from build123d import *

# Parameters (mm, degrees)
CUT_EXTRUDE1_DEPTH = 10
CIRPATTERN1_COUNT  = 20


with BuildPart() as part:
    # Sketch1 → Revolve1 (revolve)
    with BuildSketch(Plane.XY, mode=Mode.PRIVATE) as revolve1_sk:
        Polygon((0, 8), (0, 10), (7.5, 10), (7.5, 0), (4, 0), (4, 5), (3.05, 5), (3.05, 8), align=None)
    revolve(revolve1_sk.sketch.rotate(Axis((0, 0, 0), (0, 1, 0)), 90), axis=Axis((0, 0, 0), (0, 1, 0)))

    # Sketch2 → Cut-Extrude1 (cut)
    with BuildSketch(Plane(origin=(0, 10, 0), x_dir=(1, 0, 0), z_dir=(0, 1, 0))):
        Polygon((0, 8.5), (1.154700538, 8.5), (0, 6.5), (-1.154700538, 8.5), align=None)
    cut_extrude1 = extrude(amount=-CUT_EXTRUDE1_DEPTH, mode=Mode.SUBTRACT)

    # CirPattern1: Cut-Extrude1 ×20 about axis
    cirpattern1_axis = Axis((0, 0, 0), (0, 1, 0))
    for i in range(1, CIRPATTERN1_COUNT):
        add(cut_extrude1.rotate(cirpattern1_axis, i * 360 / CIRPATTERN1_COUNT), mode=Mode.SUBTRACT)

    # Sketch3 → Cut-Revolve1 (revolve, cut)
    with BuildSketch(Plane.XY):
        Polygon((-8, 8.5), (-6, 10.5), (-8, 10.5), align=None)
    revolve(axis=Axis((0, 0, 0), (0, 1, 0)), mode=Mode.SUBTRACT)


solid = part.part
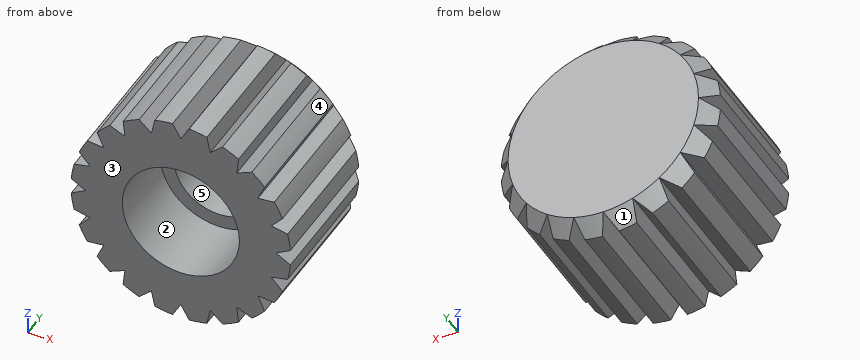
Geometry: final body of the model. Coordinates: model frame, mm. Face numbers are marked on the shaded views. A direction names the side the tool comes from. Coordinates: 2 decimals unless noted, no trailing zeros. One line per question, with ' | ' between items. Start each with the question number.
Item 1: Ray query, probe 1 along Z at (x, y) = (3.75, 5.25); probe 2 along Y at (x, z) = (2.75, -2.75); probe 3 along Z at (x, y) = (-7, 6.75). Return the intervals inside material, ascending. Write a range as [from, to].
Item 2: Pin query (flat end, axial travel): pin 1 Ø1.5 at (x, y) = (4.5, 6.5) entering from +Z; pin 2 Ø3 at (y, z) = (3.5, 4) entering from -X; pin 3 Ø4 at (x, y) = (-4, 5) entering from -Z. Return the tip coordinate at first contact, or that it passes through.
Item 3: Draft query along Z for the marked faces 3, 4 and 5. Return one class per face: released by +Z, released by -Z, zero draft, split by the parting line, or undercut.
Item 4: Set-up query: the marked faces 1 and 2. Return all of +Z, -Z, +X, -X, +Y, -Y with unobstructed straight access to the full face (end or side cutting, diameter ignored); none if empty.
Item 5: Cut plane A-A, the plane z = 5.5. Count the separate pieces of the cut face and the enclosed holes in it, then the cut area to 3 significant figures.
A:
1) probe 1: z = [-6.5, 6.5] | probe 2: y = [5, 10] | probe 3: z = [-1.83, -0.29], [0.29, 1.83]
2) pin 1: stops at z = 6.5 | pin 2: stops at x = -6.94 | pin 3: stops at z = -6.94
3) face 3: zero draft | face 4: released by +Z | face 5: undercut
4) face 1: -Z, -X, +Y | face 2: -Y
5) separate pieces: 3 | enclosed holes: 0 | area: 90.5 mm2
